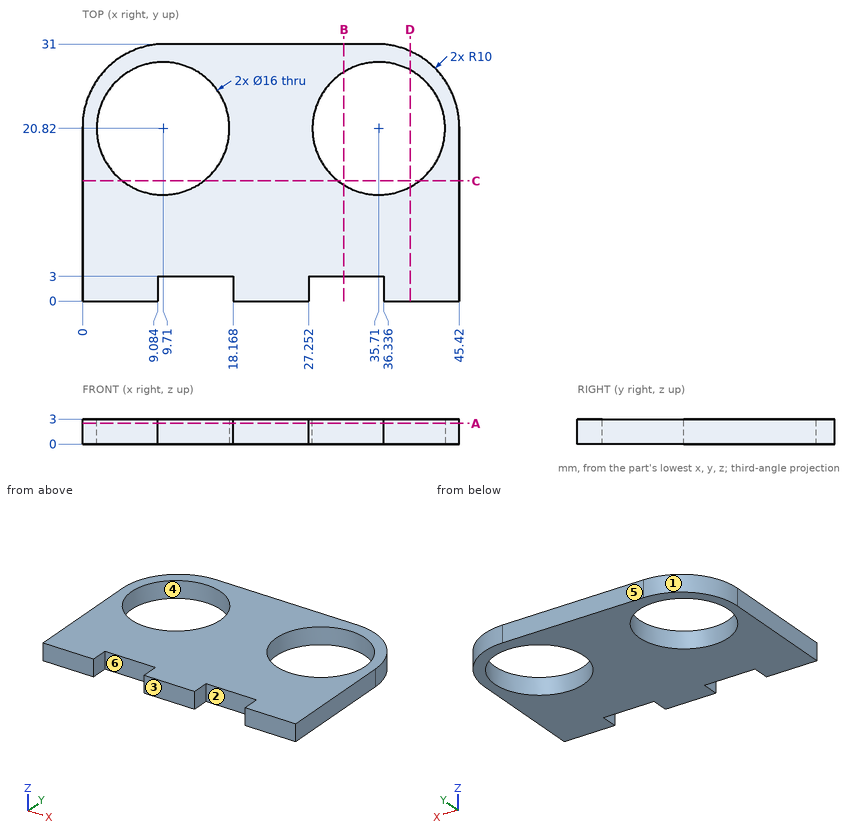
Geometry check sheet. Reference: drawing and pictorial views, mm from the part's lowest x, y, z. A direction names the side the tool comes from. Give positions to 0.01 mm unless a question says otherwise; leave off trailing zeros. Write each loop counter-clockwise with the first axis right and the second up, starting at its lowest first coordinate (ties: lowest second). Pieces come first, ordered by that corner, then holes. Notation, with made-up numbers: (-14, -18) - (42, -18) arc R27 ccw to (42, 10) - close; hole circle Ø3 at (59, 54.5). An arc over 180 degrees is marked (long way). Put each result on its own line as item: value.
Q1. Depth check by flat-ended pin: P1, Ø6, axis at x = 6, y = 23.5, coming from the -Z side; P2, Ø0.9, axis at x = 12, z = 2, coming from the -Y side. Enter the tip coordinate at first touch or a pass-through.
Result:
P1: through
P2: y = 3
Q2. Section check B-B on x = 31.5. Record the cut outline in (y, z), and give its area (3 significant figures).
Result:
outline: (3, 0) - (14.02, 0) - (14.02, 3) - (3, 3) - close; (27.62, 0) - (31, 0) - (31, 3) - (27.62, 3) - close
area: 43.2 mm2
Q3. Section check D-D on x = 39.5. Record the cut outline in (y, z), and give its area (3 significant figures).
Result:
outline: (0, 0) - (13.77, 0) - (13.77, 3) - (0, 3) - close; (27.87, 0) - (30.13, 0) - (30.13, 3) - (27.87, 3) - close
area: 48.1 mm2
Q4. Set-up check for the marked faces 5 and 6: record each of +Z, -Z, +X, -X, +Y, -Y from which the full face is reachable in a straight line by a thin tool's end or side.
Result:
face 5: +Z, -Z, +X, -X, +Y
face 6: +Z, -Z, -Y
Q5. Mould release check, pull along X, two halves, no side actions. Record for the marked faces 1, 2, 3 and 4: released by +X, released by -X, zero draft, split by the parting line, or undercut.
Result:
face 1: released by -X
face 2: undercut
face 3: zero draft
face 4: undercut
Q6. Section check A-A on z = 2.5. Record the cut outline in (x, y).
Result:
outline: (0, 0) - (9.08, 0) - (9.08, 3) - (18.17, 3) - (18.17, 0) - (27.25, 0) - (27.25, 3) - (36.34, 3) - (36.34, 0) - (45.42, 0) - (45.42, 21) arc R10 ccw to (35.42, 31) - (10, 31) arc R10 ccw to (0, 21) - close; hole circle Ø16 at (9.71, 20.82); hole circle Ø16 at (35.71, 20.82)
Q7. Section check C-C on y = 14.5. Record the cut outline in (x, z).
Result:
outline: (0, 0) - (4.81, 0) - (4.81, 3) - (0, 3) - close; (14.61, 0) - (30.81, 0) - (30.81, 3) - (14.61, 3) - close; (40.61, 0) - (45.42, 0) - (45.42, 3) - (40.61, 3) - close
Q8. Scan lines: probe 1 along Y at (x, z) = (35.71, 2.1); probe 2 along X at (y, z) = (27, 2.85); probe 3 along X at (y, z) = (17, 1.4). Record each from-to range of solid material in increasing order. Write a range as from..to.
Result:
probe 1: 3..12.82, 28.82..31
probe 2: 2..4.63, 14.79..30.63, 40.79..43.42
probe 3: 0..2.68, 16.74..28.68, 42.74..45.42
